from build123d import *

# Parameters (mm, degrees)
SKETCH_1_R               = 12
SKETCH_1_R_2             = 10.75
RING_DEPTH               = 5
SKETCH_2_W               = 50
SKETCH_2_H               = 5
STICK_DEPTH              = 5
SKETCH_3_W               = 21
SKETCH_3_H               = 5
KEY_DEPTH                = 10
FILLET_1_R               = 5
FILLET_5_R               = 3
CUT_EXTRUDE_1_DEPTH      = 63.839058045
CUT_EXTRUDE_1_DEPTH_BACK = 63.839058045


with BuildPart() as part:
    # Эскиз1 → ring (new body)
    with BuildSketch(Plane(origin=(0, 0, 0), x_dir=(1, 0, 0), z_dir=(0, 1, 0))):
        with Locations(Location((0, 0, 0), (0, 0, 270))):
            Circle(SKETCH_1_R)
        with Locations(Location((0, 0, 0), (0, 0, 270))):
            Circle(SKETCH_1_R_2, mode=Mode.SUBTRACT)
    extrude(amount=RING_DEPTH)

    # Эскиз2 → stick (add)
    with BuildSketch(Plane(origin=(0, 0, 0), x_dir=(1, 0, 0), z_dir=(0, 1, 0))):
        with Locations((-36.22497216, 0)):
            Rectangle(SKETCH_2_W, SKETCH_2_H)
    extrude(amount=STICK_DEPTH)

    # Эскиз3 → key (add)
    with BuildSketch(Plane(origin=(0, 0, 0), x_dir=(1, 0, 0), z_dir=(0, 1, 0))):
        with Locations((-50.72497216, 0)):
            Rectangle(SKETCH_3_W, SKETCH_3_H)
    extrude(amount=KEY_DEPTH)

    # Скругление1
    fillet_1_edges = [part.edges().sort_by_distance(p)[0] for p in [
        (-11.736694594, 2.5, 2.5),
        (-11.736694594, 2.5, -2.5),
    ]]
    fillet(fillet_1_edges, radius=FILLET_1_R)

    # Скругление5
    fillet_5_edges = [part.edges().sort_by_distance(p)[0] for p in [
        (-40.22497216, 5, 0),
    ]]
    fillet(fillet_5_edges, radius=FILLET_5_R)

    # Эскиз4 → Вытянуть1 (cut, two sides: drawn at the far end of the back side and taken through both)
    with BuildSketch(Plane(origin=(0, 2.5, 0), x_dir=(1, 0, 0), z_dir=(0, 1, 0)).offset(-CUT_EXTRUDE_1_DEPTH_BACK)):
        Polygon((-61.22497216, 0.5), (-41.22497216, 0.5), (-41.22497216, -0.5), (-42.388207879, -0.5), (-42.82497216, -1.7), (-44.62497216, -1.7), (-45.061736441, -0.5), (-46.22497216, -0.5), (-47.388207879, -0.5), (-47.82497216, -1.7), (-49.62497216, -1.7), (-50.061736441, -0.5), (-51.22497216, -0.5), (-52.388207879, -0.5), (-52.82497216, -1.7), (-54.62497216, -1.7), (-55.061736441, -0.5), (-56.22497216, -0.5), (-57.388207879, -0.5), (-57.82497216, -1.7), (-59.62497216, -1.7), (-60.061736441, -0.5), (-61.22497216, -0.5), align=None)
    extrude(amount=CUT_EXTRUDE_1_DEPTH + CUT_EXTRUDE_1_DEPTH_BACK, mode=Mode.SUBTRACT)


solid = part.part
Input: part model. Units: mm. Frame: model coordinates. A direction names the side the tool comes from. Give positions to 0.01 mm unless a question says otherwise; leave off trailing zeros. Write each loop counter-clockwise with the first axis right and the second up, starting at its lowest first coordinate (ties: lowest second). Pieces come first, ordered by that corner, then holes. Notation, with made-up numbers: M 9,14 L 34,14 A12 ccw 34,23 Z; hole C 15.25,38 d5. An arc over 180 degrees is marked long. Use one line per item in the form item = value.
1. Ray query, L1, parallel to X at y = 1.4, z = 0; L2, parallel to Z at x = -46, y = 9; L3, parallel to Z at x = -41, y = 5. Return the intervals inside material, ascending.
Outcome:
L1 = -41.22 to -10.75, 10.75 to 12
L2 = -2.5 to -0.5, 0.5 to 2.5
L3 = -2.5 to 2.5
2. Cut plane A-A on x = 0. Return loops of the section in (y, z).
Outcome:
outline = M 0,-12 L 5,-12 L 5,-10.75 L 0,-10.75 Z; M 0,10.75 L 5,10.75 L 5,12 L 0,12 Z
3. First-contact query: P1, Ø1.2, axis at x = -56, y = 3.5, coming from the -Z side; P2, Ø1, axis at y = 6.5, z = 7, coming from the -X side (3 decimals); P3, Ø5, axis at x = -39, y = 4.5, coming from the +Z side; P4, Ø7, axis at x = -15, z = -3, coming from the +Y side. Flat tips, straight axial feed; report the tip coordinate or a pass-through.
Outcome:
P1 = -2.5
P2 = through
P3 = 2.5
P4 = 5
4. Cut plane B-B on z = 6. Return loops of the section in (x, y), and give its area (3 significant figures).
Outcome:
outline = M -10.39,0 L -8.92,0 L -8.92,5 L -10.39,5 Z; M 8.92,0 L 10.39,0 L 10.39,5 L 8.92,5 Z
area = 14.7 mm²
5. Cut plane D-D on x = -13.5. Return loops of the section in (y, z).
Outcome:
outline = M 0,-2.82 L 5,-2.82 L 5,2.82 L 0,2.82 Z
6. Cut plane C-C on x = -29. Return loops of the section in (y, z), and give its area (3 significant figures).
Outcome:
outline = M 0,-2.5 L 5,-2.5 L 5,2.5 L 0,2.5 Z
area = 25.0 mm²
7. Mould query, pull axis Z, two halves, no side actions, for faces 1 (the face through (-39.323, 5.855, 0.035)), 2 (the face through (-59, 5, 1.7)), 3 (the face through (12, 2, 0)). Classes: released by +Z, released by -Z, zero draft, split by the parting line, or undercut.
Outcome:
face_1 = zero draft
face_2 = undercut
face_3 = split by the parting line
8. Reachability of faces 4 (the face through (-51, 5, 0.5)), 5 (the face through (-44.84, 4.93, 1.11)), 6 (the face through (-44, 4, 2.5)), 7 (the face through (-13, 5, 0)), 8 (the face through (-51, 10, -1)) from +Z, -Z, +X, -X, +Y, -Y: full face, straight path, thin tool, end or side. Return the list, or none.
Outcome:
face_4 = -X, +Y, -Y
face_5 = +Y, -Y
face_6 = +Z, -X, +Y, -Y
face_7 = +Z, -Z, +X, +Y
face_8 = +Z, -Z, +X, -X, +Y
